Geometry check sheet. Reference: drawing and pictorial views, mm from the part's lowest x, y, z. A direction names the side the tool comes from. Coordinates: 2 decimals unless noted, no trailing zeros. Order: outer loops, then holes, each group sorted by start corner. A loop starts at its lowest first (then second) coordinate and runs counter-clockwise, first axis right, second up. Notation, with made-up numbers: (-8, 47.25) -> (30, 47.25) arc R28 cw to (30, 67.25) -> close; hole circle Ø4 at (34, -26.5). An arc over 180 degrees is marked (long way). Use CSV: the item, a comma, the result in double quotes. Start each with the question number.
1) Sectioned sample at D-D on y = 77. Record the boundary of the cut face in (x, z) (1 decimal), then the cut area to 3 significant figures.
2) Sectioned sample at A-A on x = 51. Record the boundary of the cut face in (y, z) (1 decimal).
3) Scan lines: line 1 along Y through (x, z) = (68, 5.75) (1 decimal); line 2 along X through (y, z) = (40.5, 3.25) (1 decimal); line 3 along Y through (x, z) = (25.5, 11.25) (1 decimal). Record each from-to range of solid material in increasing order.
4) Sectioned sample at B-B on z = 8.75. Give the number of separate pieces and of enclosed holes in the cut face, then the cut area to 3 significant figures.
5) Sectioned sample at C-C on x = 17. Record the boundary of the cut face in (y, z) (1 decimal).
6) Release check for a two-part mould opening along X. For the marked faces 1, 2 and 3 record: released by +X, released by -X, zero draft, split by the parting line, or undercut.
7) Go/stop test with flat-tipped pins: pin 1 (4 mm diameter, centred on x = 63, z = 10.5, fed in from +Y); pin 2 (1 mm diameter, centred on x = 65, z = 3.5, fed in from +Y); pin 3 (6.5 mm diameter, centred on x = 39, y = 66, fed in from +Z). Record where each tip stops, or that it passes through.
8) Tool access check on the marked faces 4 and 5. Record the directions out of +Z, -Z, +X, -X, +Y, -Y that give a thin tool (end or side, any length) a straight path to the whole face; none if there is none.
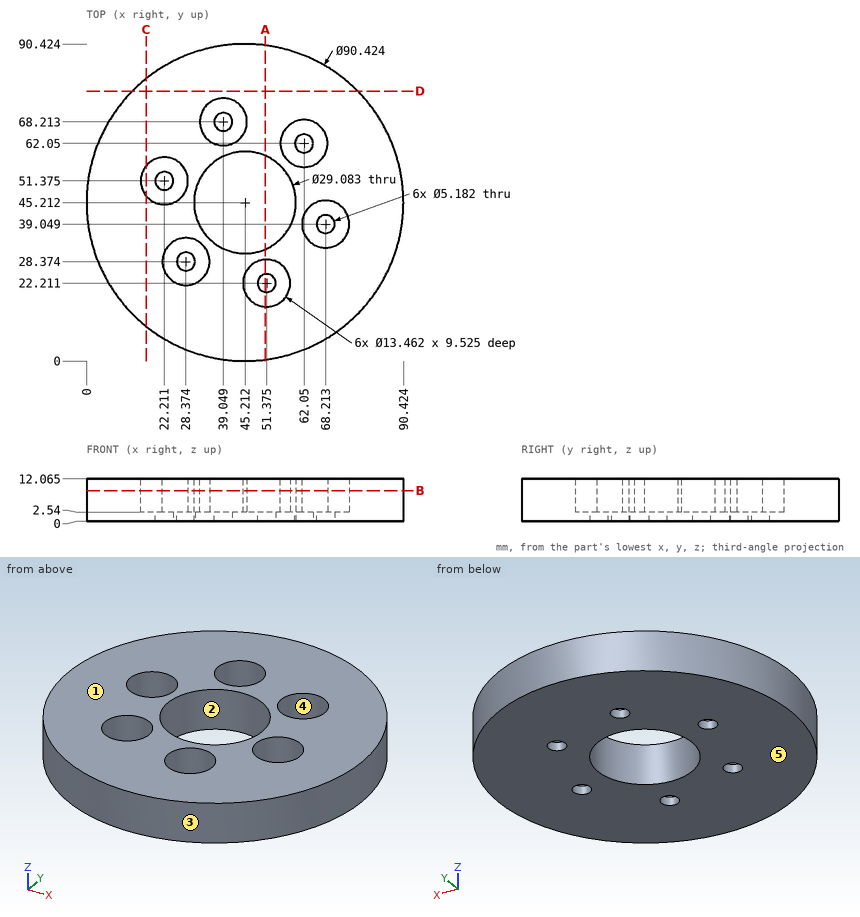
Answers follow:
1,outline,"(13.1, 0) -> (77.4, 0) -> (77.4, 12.1) -> (13.1, 12.1) -> close"
1,area,"776 mm²"
2,outline,"(0.4, 0) -> (19.6, 0) -> (19.6, 2.5) -> (15.5, 2.5) -> (15.5, 12.1) -> (0.4, 12.1) -> close; (24.8, 0) -> (31.9, 0) -> (31.9, 12.1) -> (28.9, 12.1) -> (28.9, 2.5) -> (24.8, 2.5) -> close; (58.6, 0) -> (90.1, 0) -> (90.1, 12.1) -> (58.6, 12.1) -> close"
3,line 1,"y = 6.2 to 32.3, 45.8 to 58.9, 65.2 to 84.3"
3,line 2,"x = 0.2 to 31.5, 59 to 61.6, 74.8 to 90.2"
3,line 3,"y = 4.5 to 22.3, 34.5 to 45.5, 57.2 to 85.9"
4,separate pieces,"1"
4,enclosed holes,"7"
4,area,"4,900 mm²"
5,outline,"(9.9, 0) -> (80.5, 0) -> (80.5, 12.1) -> (55.6, 12.1) -> (55.6, 2.5) -> (47.1, 2.5) -> (47.1, 12.1) -> (9.9, 12.1) -> close"
6,face 1,"zero draft"
6,face 2,"undercut"
6,face 3,"split by the parting line"
7,pin 1,"stops at y = 87.58"
7,pin 2,"stops at y = 86.1"
7,pin 3,"stops at z = 2.54"
8,face 4,"+Z"
8,face 5,"-Z, +X, -X, +Y, -Y"
